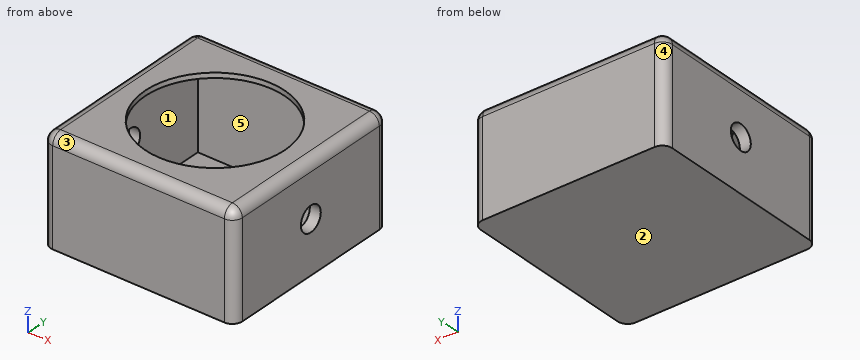
```python
from build123d import *

# Parameters (mm, degrees)
SKETCH_W        = 19.2
SKETCH_H        = 19.2
PAD_DEPTH       = 10.6
SKETCH001_R     = 1.25
POCKET_DEPTH    = 19.201
SKETCH002_R     = 7
POCKET001_DEPTH = 0.5
SKETCH003_W     = 17
SKETCH003_H     = 17
POCKET002_DEPTH = 10
FILLET_R        = 1


with BuildPart() as part:
    # Sketch → Pad (new body)
    with BuildSketch(Plane.XY):
        Rectangle(SKETCH_W, SKETCH_H)
    extrude(amount=PAD_DEPTH)

    # Sketch001 (on Face2 of Pad) → Pocket (cut, through all)
    with BuildSketch(Plane.YZ.offset(9.6)):
        with Locations((0, 5.25)):
            Circle(SKETCH001_R)
    extrude(amount=-POCKET_DEPTH, mode=Mode.SUBTRACT)

    # Sketch002 (on Face5 of Pocket) → Pocket001 (cut)
    with BuildSketch(Plane.XY.offset(10.6)):
        Circle(SKETCH002_R)
    extrude(amount=-POCKET001_DEPTH, mode=Mode.SUBTRACT)

    # Sketch003 (on Face9 of Pocket001) → Pocket002 (cut)
    with BuildSketch(Plane.XY.offset(10.1)):
        Rectangle(SKETCH003_W, SKETCH003_H)
    extrude(amount=-POCKET002_DEPTH, mode=Mode.SUBTRACT)

    # Fillet
    fillet_edges = [part.edges().sort_by_distance(p)[0] for p in [
        (9.6, -9.6, 5.3),
        (-9.6, -9.6, 5.3),
        (9.6, 9.6, 5.3),
        (-9.6, 9.6, 5.3),
        (0, -9.6, 10.6),
        (-9.6, 0, 10.6),
        (0, 9.6, 10.6),
        (9.6, 0, 10.6),
    ]]
    fillet(fillet_edges, radius=FILLET_R)


solid = part.part
```
Design review of the part built by this model. Coordinates are the model's own, in mm. Face numbers are marked on the shaded views. A direction names the side the tool comes from. Round coordinates to 2 decimals unless told otherwise and drop trailing zeros. Write each loop counter-clockwise with the first axis right and the second up, starting at its lowest first coordinate (ties: lowest second). Pieces come first, ordered by that corner, then holes. Notation, with made-up numbers: (55, 58.5) -> (80, 58.5) arc R19 ccw to (80, 76.5) -> close; hole circle Ø3 at (58.25, 35.5). An arc over 180 degrees is marked (long way). Answer in a Markdown table with one row per item.
Q1. Draft analysis for pull direction Y (two halves, no side actions). For the marked faces 3, 4 and 5, state which applies: +Y half, -Y half, draft (parallel to the pull), parting line (faces both ways), or undercut.
The answers:
| item | result |
|---|---|
| face 3 | -Y half |
| face 4 | +Y half |
| face 5 | undercut |
Q2. Clearance check with a flat-ended pin moving along its axis: pin 1 Ø1.5 at (y, z) = (0, 5.25) entering from -X. State where the tip first meets the part, or that it passes through.
The answers:
| item | result |
|---|---|
| pin 1 | through |
Q3. Take a section at B-B, the plane z = 5.25. State the section outline as (x, y) points, then the cut area to 3 significant figures.
The answers:
| item | result |
|---|---|
| outline | (-9.6, -8.6) arc R1 ccw to (-8.6, -9.6) -> (8.6, -9.6) arc R1 ccw to (9.6, -8.6) -> (9.6, -1.25) -> (8.5, -1.25) -> (8.5, -8.5) -> (-8.5, -8.5) -> (-8.5, -1.25) -> (-9.6, -1.25) -> close; (-9.6, 1.25) -> (-8.5, 1.25) -> (-8.5, 8.5) -> (8.5, 8.5) -> (8.5, 1.25) -> (9.6, 1.25) -> (9.6, 8.6) arc R1 ccw to (8.6, 9.6) -> (-8.6, 9.6) arc R1 ccw to (-9.6, 8.6) -> close |
| area | 73.3 mm² |
Q4. For the marked faces 1 and 2, list the 3-axis set-ups (+Z, -Z, +X, -X, +Y, -Y) from which the entire face can be reached by the end or side of a thin tool; tool diameter is ignored.
The answers:
| item | result |
|---|---|
| face 1 | none |
| face 2 | -Z, +X, -X, +Y, -Y |
Q5. To check wall thickness, follow L1, parallel to X at y = 3, z = 8.75; L2, parallel to Y at x = 0, z = 10.2. State the ranges of each line that lie inside material, in increasing order. Write a range as [from, to].
The answers:
| item | result |
|---|---|
| L1 | [-9.6, -8.5], [8.5, 9.6] |
| L2 | [-9.4, -7], [7, 9.4] |
Q6. Take a section at A-A, the plane y = 0. State the section outline as (x, z) points, then the cut area to 3 significant figures.
The answers:
| item | result |
|---|---|
| outline | (-9.6, 0) -> (9.6, 0) -> (9.6, 4) -> (8.5, 4) -> (8.5, 0.1) -> (-8.5, 0.1) -> (-8.5, 4) -> (-9.6, 4) -> close; (-9.6, 6.5) -> (-8.5, 6.5) -> (-8.5, 10.1) -> (-7, 10.1) -> (-7, 10.6) -> (-8.6, 10.6) arc R1 ccw to (-9.6, 9.6) -> close; (7, 10.1) -> (8.5, 10.1) -> (8.5, 6.5) -> (9.6, 6.5) -> (9.6, 9.6) arc R1 ccw to (8.6, 10.6) -> (7, 10.6) -> close |
| area | 20.6 mm² |
Q7. Take a section at D-D, the plane x = 0. State the section outline as (y, z) points, then the cut area to 3 significant figures.
The answers:
| item | result |
|---|---|
| outline | (-9.6, 0) -> (9.6, 0) -> (9.6, 9.6) arc R1 ccw to (8.6, 10.6) -> (7, 10.6) -> (7, 10.1) -> (8.5, 10.1) -> (8.5, 0.1) -> (-8.5, 0.1) -> (-8.5, 10.1) -> (-7, 10.1) -> (-7, 10.6) -> (-8.6, 10.6) arc R1 ccw to (-9.6, 9.6) -> close |
| area | 26.1 mm² |
Q8. Take a section at C-C, the plane y = 8.25. State the section outline as (x, z) points.
The answers:
| item | result |
|---|---|
| outline | (-9.6, 0) -> (9.6, 0) -> (9.6, 9.6) arc R1 ccw to (8.6, 10.6) -> (-8.6, 10.6) arc R1 ccw to (-9.6, 9.6) -> close; hole (-8.5, 0.1) -> (8.5, 0.1) -> (8.5, 10.1) -> (-8.5, 10.1) -> close |
